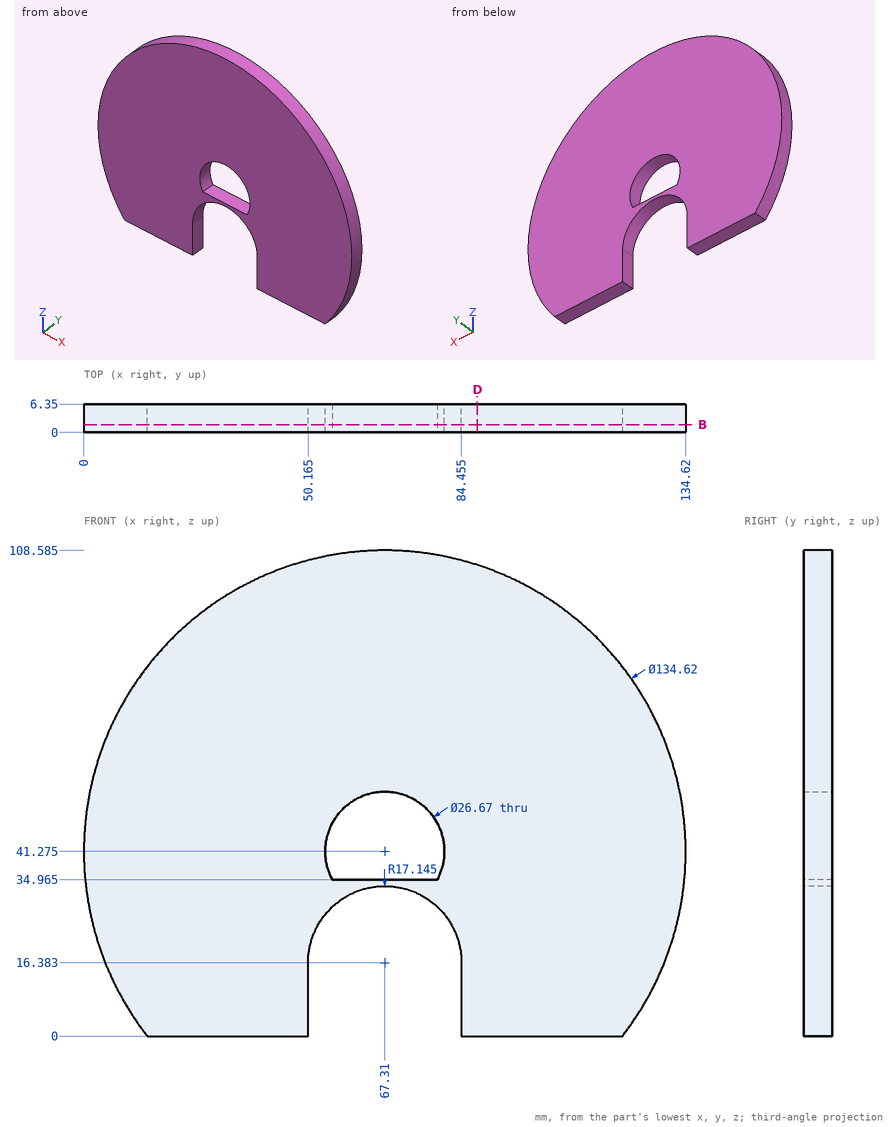
Design review of the part shown in the three views and the two pictorial views. Dimensions are in mm from the part's minimum x, y and z. Round coordinates to 2 decimals unless told otherwise and drop trailing zeros. Loops run counter-clockwise (first coordinate to the right, second up) from the corner with the lowest first, then second, coordinate; pieces in that order, holes last.
1) Wall thickness on line 1 along X through (y, z) = (5, 26.5); line 2 along Z through (x, y) = (79, 2.5) (1 decimal); line 3 along Z through (x, y) = (60.5, 2) (1 decimal): over which ranges is each line inside the solid? List them lowest first.
Values follow:
line 1: x = 1.64 to 53.47, 81.15 to 132.98
line 2: z = 28.9 to 35, 47.7 to 107.6
line 3: z = 32.1 to 35, 52.7 to 108.2
2) Consider section B-B on y = 1.75. State the section outline as (x, z) points (1 decimal), then the cut area to 3 significant figures.
Values follow:
outline: (14.1, 0) - (50.2, 0) - (50.2, 16.4) arc R17.1 cw to (84.5, 16.4) - (84.5, 0) - (120.5, 0) arc R67.3 ccw (long way) to start; hole (55.6, 35) - (79.1, 35) arc R13.3 ccw (long way) to start
area: 10,800 mm2
3) Consider section D-D on x = 88. State the section outline as (y, z) points, then the cut area to 3 significant figures.
Values follow:
outline: (0, 0) - (6.35, 0) - (6.35, 105.33) - (0, 105.33) - close
area: 669 mm2
4) Clearance check with flat-ended pins moving along their axes: P1, Ø1.9, axis at y = 4.5, z = 9, coming from the +X side; P2, Ø1.5, axis at y = 4, z = 74, coming from the -X side; P3, Ø3, axis at x = 64.5, y = 3, coming from the +Z side. State where each tip first meets the part, or that it passes through.
Values follow:
P1: stops at x = 126.89
P2: stops at x = 8.08
P3: stops at z = 108.57
